Model file for the job. Use its own axes, mm. A direction names the side the tool comes from. Give positions to 0.01 mm unless a question says otherwise; leave off trailing zeros. Write each loop counter-clockwise with the first axis right and the second up, starting at its lowest first coordinate (ties: lowest second). Pieces come first, ordered by that corner, then holes. Notation, with made-up numbers: (50, -39.75) - (55, -39.75) arc R19 ccw to (55, -24.75) - close; hole circle Ø1 at (80.5, -27). An arc over 180 degrees is marked (long way). Use a Markdown table: item, result. Add a question column.
```python
from build123d import *

# Parameters (mm, degrees)
BOSS_EXTRUDE4_DEPTH   = 41.275
BOSS_EXTRUDE4_2_DEPTH = 41.275
BOSS_EXTRUDE4_3_DEPTH = 41.275
BOSS_EXTRUDE4_4_DEPTH = 41.275
CUT_EXTRUDE12_DEPTH   = 10.668
CUT_EXTRUDE13_DEPTH   = 29.972
CUT_EXTRUDE7_DEPTH    = 44.0276
CUT_EXTRUDE9_DEPTH    = 15.24
BOSS_EXTRUDE6_DEPTH   = 5.969
CUT_EXTRUDE15_DEPTH   = 19.05
REVOLVE1_ANGLE        = 142
CUT_REVOLVE1_ANGLE    = 153
SKETCH39_W            = 642.112
SKETCH39_H            = 43.0276
BOSS_EXTRUDE5_DEPTH   = 6.35
SKETCH38_R            = 155.575
CUT_EXTRUDE14_DEPTH   = 3.429
CUT_EXTRUDE16_DEPTH   = 48.244


with BuildPart() as part:
    # Sketch5 → Boss-Extrude4 (new body)
    with BuildSketch(Plane(origin=(0, 88.9762, 0), x_dir=(1, 0, 0), z_dir=(0, 1, 0))):
        Polygon((281.7495, 153.8224), (9.144, 153.8224), (9.144, 157.3022), (14.224, 157.3022), (14.224, 167.0304), (261.323220327, 167.0304), align=None)
    extrude(amount=BOSS_EXTRUDE4_DEPTH)


with BuildPart() as body_2:
    # Sketch5 → Boss-Extrude4 2 (new body)
    with BuildSketch(Plane(origin=(0, 88.9762, 0), x_dir=(1, 0, 0), z_dir=(0, 1, 0))):
        with BuildLine():
            Line((9.144, 196.85), (230.476735197, 196.85))
            ThreePointArc((230.476735197, 196.85), (228.329031076, 193.294962827), (226.362857042, 189.6364))
            Line((226.362857042, 189.6364), (235.397557666, 183.7944))
            Line((235.397557666, 183.7944), (152.4, 183.7944))
            Line((152.4, 183.7944), (139.7, 185.8264))
            Line((139.7, 185.8264), (14.224, 185.8264))
            Line((14.224, 185.8264), (14.224, 193.3702))
            Line((14.224, 193.3702), (9.144, 193.3702))
            Line((9.144, 193.3702), (9.144, 196.85))
        make_face()
    extrude(amount=BOSS_EXTRUDE4_2_DEPTH)


with BuildPart() as body_3:
    # Sketch5 → Boss-Extrude4 3 (new body)
    with BuildSketch(Plane(origin=(0, 88.9762, 0), x_dir=(1, 0, 0), z_dir=(0, 1, 0))):
        with BuildLine():
            Line((364.677442334, 183.7944), (373.712142958, 189.6364))
            ThreePointArc((373.712142958, 189.6364), (371.745968924, 193.294962827), (369.598264803, 196.85))
            Line((369.598264803, 196.85), (651.256, 196.85))
            Line((651.256, 196.85), (651.256, 193.3702))
            Line((651.256, 193.3702), (646.176, 193.3702))
            Line((646.176, 193.3702), (646.176, 185.8264))
            Line((646.176, 185.8264), (460.375, 185.8264))
            Line((460.375, 185.8264), (447.675, 183.7944))
            Line((447.675, 183.7944), (364.677442334, 183.7944))
        make_face()
    extrude(amount=BOSS_EXTRUDE4_3_DEPTH)


with BuildPart() as body_4:
    # Sketch5 → Boss-Extrude4 4 (new body)
    with BuildSketch(Plane(origin=(0, 88.9762, 0), x_dir=(1, 0, 0), z_dir=(0, 1, 0))):
        Polygon((646.176, 167.0304), (338.751779673, 167.0304), (318.3255, 153.8224), (651.256, 153.8224), (651.256, 157.3022), (646.176, 157.3022), align=None)
    extrude(amount=BOSS_EXTRUDE4_4_DEPTH)


with BuildPart() as cut_extrude12_tool:
    # Sketch22<2> → Cut-Extrude12 (new body)
    with BuildSketch(Plane.XY.offset(-153.8224)):
        Polygon((318.3255, 96.926341572), (384.316635768, 130.2512), (215.758364232, 130.2512), (281.7495, 96.926341572), (281.7495, 92.1512), (318.3255, 92.1512), align=None)
    extrude(amount=-CUT_EXTRUDE12_DEPTH)


with BuildPart() as part_1:
    add(part.part)

    # Cut-Extrude12: cut by cut_extrude12_tool
    add(cut_extrude12_tool.part, mode=Mode.SUBTRACT)


with BuildPart() as body_4_1:
    add(body_4.part)

    # Cut-Extrude12: cut by cut_extrude12_tool
    add(cut_extrude12_tool.part, mode=Mode.SUBTRACT)


with BuildPart() as cut_extrude13_tool:
    # Sketch22<3> → Cut-Extrude13 (new body)
    with BuildSketch(Plane.XY.offset(-153.8224)):
        Polygon((318.3255, 96.926341572), (384.316635768, 130.2512), (215.758364232, 130.2512), (281.7495, 96.926341572), (281.7495, 92.1512), (318.3255, 92.1512), align=None)
    extrude(amount=-CUT_EXTRUDE13_DEPTH)


with BuildPart() as part_2:
    add(part_1.part)

    # Cut-Extrude13: cut by cut_extrude13_tool
    add(cut_extrude13_tool.part, mode=Mode.SUBTRACT)


with BuildPart() as body_4_2:
    add(body_4_1.part)

    # Cut-Extrude13: cut by cut_extrude13_tool
    add(cut_extrude13_tool.part, mode=Mode.SUBTRACT)

    # Sketch26 → Cut-Extrude9 (cut)
    with BuildSketch(Plane.XY.offset(-153.8224)):
        Polygon((510.032, 130.2512), (505.206, 125.4252), (474.218, 125.4252), (467.106, 118.3132), (396.254635768, 118.3132), (384.316635768, 130.2512), align=None)
    extrude(amount=-CUT_EXTRUDE9_DEPTH, mode=Mode.SUBTRACT)


with BuildPart() as cut_extrude7_tool:
    # Sketch22 → Cut-Extrude7 (new body, through all)
    with BuildSketch(Plane.XY.offset(-153.8224)):
        Polygon((318.3255, 96.926341572), (384.316635768, 130.2512), (215.758364232, 130.2512), (281.7495, 96.926341572), (281.7495, 92.1512), (318.3255, 92.1512), align=None)
    extrude(amount=-CUT_EXTRUDE7_DEPTH)


with BuildPart() as body_2_1:
    add(body_2.part)

    # Cut-Extrude7: cut by cut_extrude7_tool
    add(cut_extrude7_tool.part, mode=Mode.SUBTRACT)



with BuildPart() as body_3_1:
    add(body_3.part)

    # Cut-Extrude7: cut by cut_extrude7_tool
    add(cut_extrude7_tool.part, mode=Mode.SUBTRACT)

    # Sketch42 → Boss-Extrude6 (add)
    with BuildSketch(Plane(origin=(0, 130.2512, 0), x_dir=(1, 0, 0), z_dir=(0, 1, 0))):
        Polygon((396.254635768, 196.85), (510.032, 196.85), (510.032, 185.8264), (460.375, 185.8264), (447.675, 183.7944), (396.254635768, 183.7944), align=None)
    extrude(amount=BOSS_EXTRUDE6_DEPTH)

    # Sketch36 → Cut-Extrude15 (cut)
    with BuildSketch(Plane.XY.offset(-196.85)):
        Polygon((435.356, 117.4242), (454.2028, 136.271), (477.819866452, 136.271), (492.506, 121.584866452), (501.365666452, 121.584866452), (510.032, 130.2512), (531.547497997, 151.766697997), (332.480700093, 151.766697997), (332.480700093, 117.4242), align=None)
    extrude(amount=CUT_EXTRUDE15_DEPTH, mode=Mode.SUBTRACT)


with BuildPart() as body_2_2:
    add(body_2_1.part)

    add(body_3_1.part)  # Revolve1 merges body 3
    # Sketch37 → Revolve1 (revolve, symmetric)
    with BuildSketch(Plane(origin=(300.0502, 0, 0), x_dir=(0, 0, -1), z_dir=(1, 0, 0))) as revolve1_sk:
        Polygon((238.506, 88.9762), (285.242, 88.9762), (285.242, 117.4242), (267.462, 117.4242), align=None)
    revolve(axis=Axis((300.0502, 133.091662173, -152.4), (0, -1, 0)), revolution_arc=REVOLVE1_ANGLE / 2)
    revolve(revolve1_sk.sketch, axis=Axis((300.0502, 133.091662173, -152.4), (0, 1, 0)), revolution_arc=REVOLVE1_ANGLE / 2)


with BuildPart() as cut_revolve1_tool:
    # Sketch41 → Cut-Revolve1 (revolve, symmetric)
    with BuildSketch(Plane(origin=(300.0502, 0, 0), x_dir=(0, 0, -1), z_dir=(1, 0, 0))) as cut_revolve1_sk:
        Polygon((290.213142857, 139.7762), (238.506, 88.9762), (171.45, 88.9762), (171.45, 139.7762), align=None)
    revolve(axis=Axis((300.0502, 150.973417034, -152.4), (0, -1, 0)), revolution_arc=CUT_REVOLVE1_ANGLE / 2)
    revolve(cut_revolve1_sk.sketch, axis=Axis((300.0502, 150.973417034, -152.4), (0, 1, 0)), revolution_arc=CUT_REVOLVE1_ANGLE / 2)


with BuildPart() as part_3:
    add(part_2.part)

    # Cut-Revolve1: cut by cut_revolve1_tool
    add(cut_revolve1_tool.part, mode=Mode.SUBTRACT)



with BuildPart() as body_2_3:
    add(body_2_2.part)

    # Cut-Revolve1: cut by cut_revolve1_tool
    add(cut_revolve1_tool.part, mode=Mode.SUBTRACT)


with BuildPart() as body_4_3:
    add(body_4_2.part)

    # Cut-Revolve1: cut by cut_revolve1_tool
    add(cut_revolve1_tool.part, mode=Mode.SUBTRACT)


with BuildPart() as part_4:
    add(part_3.part)

    add(body_2_3.part)  # Boss-Extrude5 merges body 2

    add(body_4_3.part)  # Boss-Extrude5 merges body 4
    # Sketch39 → Boss-Extrude5 (add)
    with BuildSketch(Plane.XZ.offset(-88.9762)):
        with Locations((330.2, -175.3362)):
            Rectangle(SKETCH39_W, SKETCH39_H)
    extrude(amount=-BOSS_EXTRUDE5_DEPTH)

    # Sketch38 → Cut-Extrude14 (cut)
    with BuildSketch(Plane.XZ.offset(-88.9762)):
        with Locations((300.0502, -152.4)):
            Circle(SKETCH38_R)
    extrude(amount=-CUT_EXTRUDE14_DEPTH, mode=Mode.SUBTRACT)

    # Sketch43 → Cut-Extrude16 (cut, through all)
    with BuildSketch(Plane(origin=(0, 136.2202, 0), x_dir=(1, 0, 0), z_dir=(0, 1, 0))):
        with BuildLine():
            Line((281.7495, 153.8224), (222.257640496, 196.85))
            ThreePointArc((222.257640496, 196.85), (300.0502, 241.996232143), (377.842759504, 196.85))
            Line((377.842759504, 196.85), (318.3255, 153.8224))
            Line((318.3255, 153.8224), (281.7495, 153.8224))
        make_face()
    extrude(amount=-CUT_EXTRUDE16_DEPTH, mode=Mode.SUBTRACT)


solid = part_4.part
```
(1) Which spindle directions (+Z, -Z, +X, -X, +Y, -Y) get a long thin tool onto all of the face, cutting with end or side? Do faces 1 (the flat face through (175, 109, -183.794)), 2 (the flat face through (490, 125.425, -160)), 3 (the flat face through (252.42, 93.886, -175.035)). Say none if no direction does.
(2) Probe probe 1 along Z at (x, y) = (617, 113); probe 2 along X at (y, z) = (122, -189.5); probe 3 along Z at (x, y) = (431, 112). List the from-to ranges inside material, lowest first. Write a range as [from, to].
(3) Band-saw the part on B-B (y = 107.5). Give the number of separate pieces and of enclosed holes in the cut face, then the cut area to 3 significant figures.
(4) Two-plate mould, pull along Z, no slides. Class faces 4 (the flat face through (454.114, 115.487, -184.825)), 5 (the flat face through (347.482, 104.489, -163.787)), 6 (the flat face through (485.09, 129, -191.42)), 7 (the flat face through (100, 109, -196.85)): +Z half, -Z half, draft (parallel to the pull), parting line (faces both ways), or undercut.
(5) Band-saw the part on A-A (x = 130). Write the cut outline in (y, z), then the cut area to 3 significant figures.
(6) Flat gauge pins, fed straight in: pin 1 (6.5 mm diameter, centred on x = 491.5, z = -158.5, fed in from +Y); pin 2 (10.5 mm diameter, centred on x = 514.5, y = 105.5, fed in from -Z); pin 3 (21.5 mm diameter, centred on x = 147, z = -180, fed in from +Y); pin 4 (8.5 mm diameter, centred on y = 117.5, z = -189.5, fed in from +X). Where does each tip first touch, or does it go through?
Model answer:
| question | item | result |
|---|---|---|
| 1 | face 1 | -X, +Y |
| 1 | face 2 | +Z, +Y |
| 1 | face 3 | +Y, -Y |
| 2 | probe 1 | z = [-196.85, -185.83], [-167.03, -153.82] |
| 2 | probe 2 | x = [14.22, 186.22], [439.93, 492.09], [501.78, 646.18] |
| 2 | probe 3 | z = [-196.85, -183.79], [-167.03, -153.82] |
| 3 | separate pieces | 3 |
| 3 | enclosed holes | 0 |
| 3 | area | 20,200 mm^2 |
| 4 | face 4 | undercut |
| 4 | face 5 | undercut |
| 4 | face 6 | draft |
| 4 | face 7 | -Z half |
| 5 | outline | (88.98, -196.85) - (130.25, -196.85) - (130.25, -185.83) - (95.33, -185.83) - (95.33, -167.03) - (130.25, -167.03) - (130.25, -153.82) - (88.98, -153.82) - close |
| 5 | area | 1,120 mm^2 |
| 6 | pin 1 | stops at y = 125.43 |
| 6 | pin 2 | stops at z = -196.85 |
| 6 | pin 3 | stops at y = 130.25 |
| 6 | pin 4 | stops at x = 651.26 |
